```python
from build123d import *

# Parameters (mm, degrees)
F1_DEPTH = 25
F2_R     = 12.5
F3_DEPTH = 25.001


with BuildPart() as f1:
    # F0 (on Front) → F1 (new body)
    with BuildSketch(Plane.XZ):
        Polygon((0, 50), (0, 0), (105, 0), (105, 50), (80, 50), (52.5, 22.5), (25, 50), align=None)
    extrude(amount=F1_DEPTH)

    # F2 (on face) → F3 (cut, through all)
    with BuildSketch(Plane.XZ.offset(25)):
        with Locations((20, 30)):
            Circle(F2_R)
        with Locations((85, 30)):
            Circle(F2_R)
    extrude(amount=-F3_DEPTH, mode=Mode.SUBTRACT)


solid = f1.part
```
Input: part model. Units: mm. Frame: model coordinates. A direction names the side the tool comes from. Round coordinates to 2 decimals unless told otherwise and drop trailing zeros. Order: outer loops, then holes, each group sorted by start corner. A loop starts at its lowest first (then second) coordinate and runs counter-clockwise, first axis right, second up. Notation, with made-up numbers: (49.25, 5.25) - (54.25, 5.25) arc R21 ccw to (54.25, 10.25) - close; hole circle Ø11 at (55, -0.5). An arc over 180 degrees is marked (long way). Answer in a Markdown table with one row per item.
Item 1: Mould query, pull axis Z, two halves, no side actions, for faces 1 (the flat face through (52, -12, 0)), 2 (the flat face through (52, -25, 20)), 3 (the flat face through (93, -12, 50)), 4 (the cylindrical face through (26.72, -12.68, 40.54)). Classes: released by +Z, released by -Z, zero draft, split by the parting line, or undercut.
Model answer:
| item | result |
|---|---|
| face 1 | released by -Z |
| face 2 | zero draft |
| face 3 | released by +Z |
| face 4 | undercut |
Item 2: Section query D-D (z = 30). Return the cut outline in (x, y), then the cut area to 3 significant figures.
Model answer:
| item | result |
|---|---|
| outline | (0, -25) - (7.5, -25) - (7.5, 0) - (0, 0) - close; (32.5, -25) - (45, -25) - (45, 0) - (32.5, 0) - close; (60, -25) - (72.5, -25) - (72.5, 0) - (60, 0) - close; (97.5, -25) - (105, -25) - (105, 0) - (97.5, 0) - close |
| area | 1,000 mm² |
Item 3: Section query C-C (y = -1.75). Return the cut outline in (x, z).
Model answer:
| item | result |
|---|---|
| outline | (0, 0) - (105, 0) - (105, 50) - (80, 50) - (52.5, 22.5) - (25, 50) - (0, 50) - close; hole circle Ø25 at (20, 30); hole circle Ø25 at (85, 30) |
Item 4: Section query A-A (x = 85). Return the cut outline in (y, z), then the cut area to 3 significant figures.
Model answer:
| item | result |
|---|---|
| outline | (-25, 0) - (0, 0) - (0, 17.5) - (-25, 17.5) - close; (-25, 42.5) - (0, 42.5) - (0, 50) - (-25, 50) - close |
| area | 625 mm² |
Item 5: Pin query (flat end, axial travel): pin 1 (1 mm diameter, centred on x = 28.5, z = 24.5, fed in from -Y). Return the tip coordinate at first contact, or that it passes through.
Model answer:
| item | result |
|---|---|
| pin 1 | passes through |
Item 6: Section query B-B (z = 44.5). Return the cut outline in (x, y).
Model answer:
| item | result |
|---|---|
| outline | (0, -25) - (30.5, -25) - (30.5, 0) - (0, 0) - close; (74.5, -25) - (105, -25) - (105, 0) - (74.5, 0) - close |
Item 7: Reachability of faces 5 (the flat face through (52, 0, 20)), 6 (the flat face through (66, -12, 36)) from +Z, -Z, +X, -X, +Y, -Y: full face, straight path, thin tool, end or side. Return the list, or none.
Model answer:
| item | result |
|---|---|
| face 5 | +Z, -Z, +X, -X, +Y |
| face 6 | +Z, +Y, -Y |
Item 8: Line query: line 1 (Z direction, x = 85, y = -17.75); line 2 (X direction, y = -6.25, z = 35); line 3 (X direction, y = -16, z = 38). Output: solid intervals per line, ascending.
Model answer:
| item | result |
|---|---|
| line 1 | z = 0 to 17.5, 42.5 to 50 |
| line 2 | x = 0 to 8.54, 31.46 to 40, 65 to 73.54, 96.46 to 105 |
| line 3 | x = 0 to 10.4, 29.6 to 37, 68 to 75.4, 94.6 to 105 |
